CAD build for the part. Positions are in the model's coordinates, mm. A direction names the side the tool comes from. Coordinates: 2 decimals unless noted, no trailing zeros. Write each loop counter-clockwise with the first axis right and the second up, starting at its lowest first coordinate (ties: lowest second). Pieces come first, ordered by that corner, then holes. Notation, with made-up numbers: (60, 75.25) - (65, 75.25) arc R25 cw to (65, 90.25) - close; hole circle Ø9 at (1.25, 82.5). An arc over 180 degrees is marked (long way). Answer in a Markdown table with one row per item. Add a question column.
Q1. Drill centre lines: line 1 along Y through (x, z) = (77.05, -5.4); line 2 along Z through (x, y) = (79, 55); line 3 along Y through (x, z) = (46.5, -33). Where is each one in solid material? Low to high. Write a range as from..to.
Q2. 3-axis set-ups, long thin cutter, end or side, ignore diameter. For faces 5 (the cylindrical face through (77.97, 37.92, -10.83)), 6 (the flat face through (37, 4, -29)): which of +Z, -Z, +X, -X, +Y, -Y reach the whole face in a straight line?
Q3. Pin check, flat tips, straight feed: pin 1 (1 mm diameter, centred on y = 69.5, z = -36.5, fed in from -X); pin 2 (1 mm diameter, centred on x = 17, z = -12, fed in from +Y). Stop position of each tip, or through.
Q4. Band-saw the part on A-A (y = 32.2). List the corners of the cut face in (x, z), and give its area (3 significant figures).
Q5. Band-saw the part on D-D (z = -52.6). List the corners of the cut face in (x, y).
Q6. Band-saw the part on B-B (z = -29). List the corners of the cut face in (x, y).
Q7. Band-saw the part on C-C (y = 8.6). List the corners of the cut face in (x, z).
Q8. Two-plate mould, pull along Z, no slides. Class faces 1 (the cylindrical face through (77.97, 53.31, -53.15)), 2 (the flat face through (58, 1, -58)), 3 (the flat face through (76, 50, -16)), 4 (the cylindrical face through (77.97, 53.31, -5.95)): +Z half, -Z half, draft (parallel to the pull), parting line (faces both ways), or undercut.
```python
from build123d import *

# Parameters (mm, degrees)
SKETCH1_W           = 76
SKETCH1_H           = 58
SKETCH1_W_2         = 4
BOSS_EXTRUDE1_DEPTH = 4
SKETCH1_3_W         = 4
SKETCH1_3_H         = 58
BOSS_EXTRUDE2_DEPTH = 80
SKETCH3_R           = 19.05
SKETCH3_R_2         = 2.55
CUT_EXTRUDE1_DEPTH  = 80


with BuildPart() as part:
    # Sketch1 → Boss-Extrude1 (new body)
    with BuildSketch(Plane(origin=(0, 0, 0), x_dir=(1, 0, 0), z_dir=(0, 1, 0))):
        with Locations((38, 29)):
            Rectangle(SKETCH1_W, SKETCH1_H)
        with Locations((78, 29)):
            Rectangle(SKETCH1_W_2, SKETCH1_H)
    extrude(amount=BOSS_EXTRUDE1_DEPTH)

    # Sketch1_3 → Boss-Extrude2 (add)
    with BuildSketch(Plane(origin=(0, 0, 0), x_dir=(1, 0, 0), z_dir=(0, 1, 0))):
        with Locations((78, 29)):
            Rectangle(SKETCH1_3_W, SKETCH1_3_H)
    extrude(amount=BOSS_EXTRUDE2_DEPTH)

    # Sketch3 → Cut-Extrude1 (cut)
    with BuildSketch(Plane.ZY.offset(-76)):
        with Locations((-29, 32.2)):
            Circle(SKETCH3_R)
        with Locations((-5.4, 55.8)):
            Circle(SKETCH3_R_2)
        with Locations((-52.6, 55.8)):
            Circle(SKETCH3_R_2)
        with Locations((-52.6, 8.6)):
            Circle(SKETCH3_R_2)
        with Locations((-5.4, 8.6)):
            Circle(SKETCH3_R_2)
    extrude(amount=-CUT_EXTRUDE1_DEPTH, mode=Mode.SUBTRACT)


solid = part.part
```
Checked values:
| question | item | result |
|---|---|---|
| 1 | line 1 | y = 0..6.05, 11.15..53.25, 58.35..80 |
| 1 | line 2 | z = -58..-55.02, -50.18..-7.82, -2.98..0 |
| 1 | line 3 | y = 0..4 |
| 2 | face 5 | +X, -X |
| 2 | face 6 | +Z, -Z, -X, +Y |
| 3 | pin 1 | stops at x = 76 |
| 3 | pin 2 | stops at y = 4 |
| 4 | outline | (76, -58) - (80, -58) - (80, -48.05) - (76, -48.05) - close; (76, -9.95) - (80, -9.95) - (80, 0) - (76, 0) - close |
| 4 | area | 79.6 mm² |
| 5 | outline | (0, 0) - (80, 0) - (80, 6.05) - (76, 6.05) - (76, 4) - (0, 4) - close; (76, 11.15) - (80, 11.15) - (80, 53.25) - (76, 53.25) - close; (76, 58.35) - (80, 58.35) - (80, 80) - (76, 80) - close |
| 6 | outline | (0, 0) - (80, 0) - (80, 13.15) - (76, 13.15) - (76, 4) - (0, 4) - close; (76, 51.25) - (80, 51.25) - (80, 80) - (76, 80) - close |
| 7 | outline | (76, -58) - (80, -58) - (80, -55.15) - (76, -55.15) - close; (76, -50.05) - (80, -50.05) - (80, -7.95) - (76, -7.95) - close; (76, -2.85) - (80, -2.85) - (80, 0) - (76, 0) - close |
| 8 | face 1 | undercut |
| 8 | face 2 | -Z half |
| 8 | face 3 | draft |
| 8 | face 4 | undercut |
